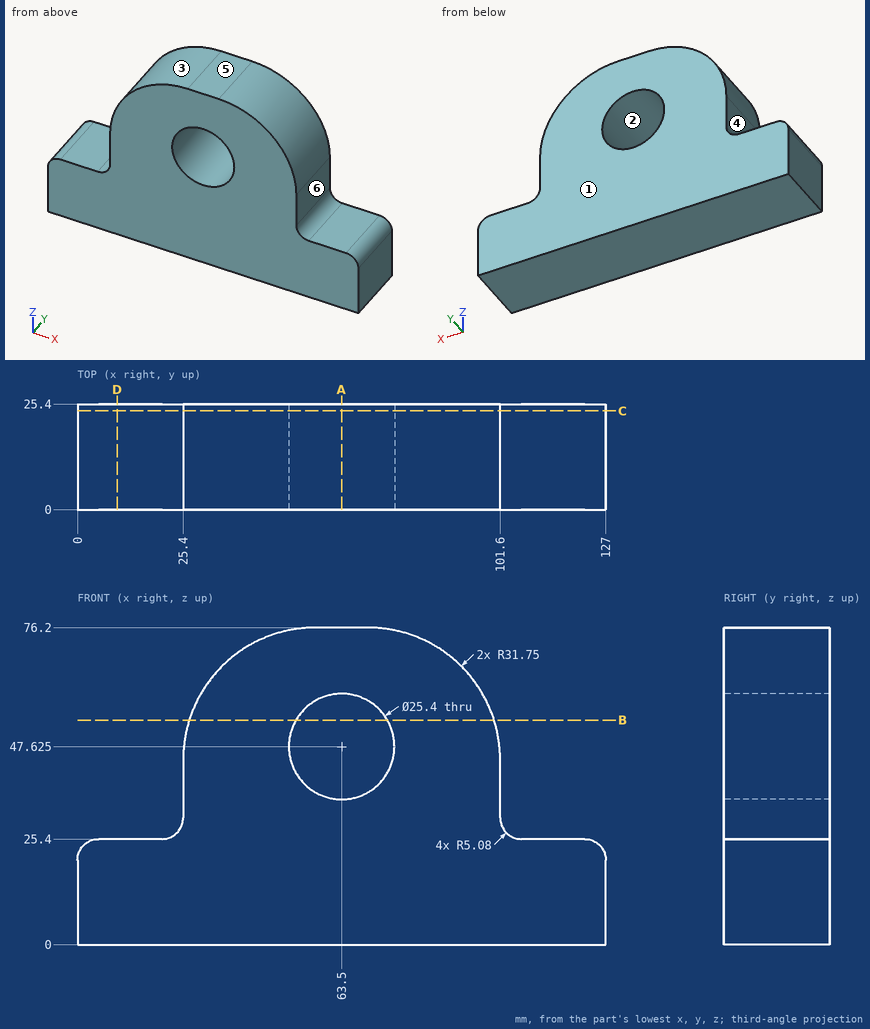
Drawing for the job (mm, zero at the part's lowest x, y, z). A direction names the side the tool comes from. Round coordinates to 2 decimals unless told otherwise and drop trailing zeros. Order: outer loops, then holes, each group sorted by start corner. A loop starts at its lowest first (then second) coordinate and runs counter-clockwise, first axis right, second up. Notation, with made-up numbers: M 2.25,77.5 L 39.25,77.5 A28 ccw 39.25,114.5 Z; hole C -5.5,25 d3. An arc over 180 degrees is marked long. Use one line per item in the form item = value.
Q1. Flat gauge pins, fed straight in: P1, Ø1.5, axis at x = 89, y = 12, coming from the +Z side; P2, Ø7, axis at y = 17.5, z = 39, coming from the -X side; P3, Ø2, axis at x = 79, y = 8.5, coming from the +Z side. Where does each tip first touch, or does it go through?
Recorded:
P1 = 70.32
P2 = 25.4
P3 = 75.14
Q2. Which spindle directions (+Z, -Z, +X, -X, +Y, -Y) get a long thin tool onto all of the face, cutting with end or side? Do the marked faces 4, 5 and 6. Say none if no direction does.
Recorded:
face_4 = +Z, -X, +Y, -Y
face_5 = +Z, +X, -X, +Y, -Y
face_6 = +Z, +X, +Y, -Y
Q3. Saw through at D-D on x = 9.5. Give the cut face in (y, z).
Recorded:
outline = M 0,0 L 25.4,0 L 25.4,25.4 L 0,25.4 Z
Q4. Two-plate mould, pull along X, no slides. Class the marked faces 1, 2 and 3: +X half, -X half, draft (parallel to the pull), parting line (faces both ways), or undercut.
Recorded:
face_1 = draft
face_2 = undercut
face_3 = -X half
Q5. Probe L1, parallel to Z at x = 63.5, y = 10.75 (3 decimals); L2, parallel to X at y = 14.25, z = 34.5; L3, parallel to X at y = 6.75, z = 46. List the from-to ranges inside material, lowest first.
Recorded:
L1 = 0 to 34.925, 60.325 to 76.2
L2 = 25.4 to 101.6
L3 = 25.44 to 50.9, 76.1 to 101.56
Q6. Saw through at B-B on z = 54. Give the cut face in (x, y), then the cut area to 3 significant figures.
Recorded:
outline = M 26.87,0 L 52.52,0 L 52.52,25.4 L 26.87,25.4 Z; M 74.48,0 L 100.13,0 L 100.13,25.4 L 74.48,25.4 Z
area = 1,300 mm^2
Q7. Saw through at A-A on x = 63.5. Give the cut face in (y, z) (3 decimals).
Recorded:
outline = M 0,0 L 25.4,0 L 25.4,34.925 L 0,34.925 Z; M 0,60.325 L 25.4,60.325 L 25.4,76.2 L 0,76.2 Z
Q8. Saw through at C-C on y = 23.75. Give the cut face in (x, z) (3 decimals), then the cut area to 3 significant figures.
Recorded:
outline = M 0,0 L 127,0 L 127,20.32 A5.08 ccw 121.92,25.4 L 106.68,25.4 A5.08 cw 101.6,30.48 L 101.6,44.45 A31.75 ccw 69.85,76.2 L 57.15,76.2 A31.75 ccw 25.4,44.45 L 25.4,30.48 A5.08 cw 20.32,25.4 L 5.08,25.4 A5.08 ccw 0,20.32 Z; hole C 63.5,47.625 d25.4
area = 6,160 mm^2
